```python
from build123d import *

# Parameters (mm, degrees)
F0_R     = 34.5
F1_DEPTH = 1
F2_R     = 34.5
F2_R_2   = 33.5
F3_DEPTH = 18
F4_R     = 40.5
F4_R_2   = 34.5
F4_R_3   = 33.5
F5_DEPTH = 1
F6_SIZE  = 0.99999
F7_R     = 2.5
F8_DEPTH = 25


# Not quite as in the source:
# - a fillet or chamfer is up to 0.001 mm smaller than in the source, because OpenCascade refuses the exact size


with BuildPart() as f1:
    # F0 (on Top) → F1 (new body)
    with BuildSketch(Plane.XY):
        Circle(F0_R)
    extrude(amount=F1_DEPTH)

    # F2 (on face) → F3 (join)
    with BuildSketch(Plane.XY.offset(1)):
        Circle(F2_R)
        Circle(F2_R_2, mode=Mode.SUBTRACT)
    extrude(amount=F3_DEPTH)

    # F4 (on face) → F5 (join)
    with BuildSketch(Plane.XY.offset(19)):
        Circle(F4_R)
        Circle(F4_R_2, mode=Mode.SUBTRACT)
        Circle(F4_R_2)
        Circle(F4_R_3, mode=Mode.SUBTRACT)
    extrude(amount=F5_DEPTH)

    # F6 (size 1 in the source; OpenCascade refuses exactly that, so slightly less here)
    f6_edges = [f1.edges().sort_by_distance(p)[0] for p in [
        (-33.5, 0, 1),
        (-34.5, 0, 0),
        (-33.5, 0, 20),
        (-40.5, 0, 20),
    ]]
    chamfer(f6_edges, length=F6_SIZE)


with BuildPart() as f8:
    # F7 (on Top) → F8 (new body)
    with BuildSketch(Plane.XY):
        with Locations((0, -33.4984026849)):
            Circle(F7_R)
    extrude(amount=F8_DEPTH)


with BuildPart() as f1_1:
    add(f1.part)

    # F9: cut F8
    add(f8.part, mode=Mode.SUBTRACT)


solid = f1_1.part
```
Work out the finished part from the listing and answer in its coordinate system (mm). Round coordinates to 2 decimals unless told otherwise and drop trailing zeros. Loops run counter-clockwise (first coordinate to the right, second up) from the corner with the lowest first, then second, coordinate; pieces in that order, holes last.
(1) The part is cut by section B-B, the plane z = 16.5. Give the vertices of the cut face in (x, y), and give its area (3 significant figures).
Computed values:
outline: (-2.5, -33.41) arc R33.5 cw (long way) to (2.5, -33.41) arc R2.5 cw to (2.32, -34.42) arc R34.5 ccw (long way) to (-2.32, -34.42) arc R2.5 cw to start
area: 209 mm2
(2) Find the intervals of material crossed by L1, parallel to X at y = 0, z = 13.5; L2, parallel to Y at x = 0, z = 11; L3, parallel to X at y = -27.5, z = 8.5, in increasing order.
Computed values:
L1: x = -34.5 to -33.5, 33.5 to 34.5
L2: y = 33.5 to 34.5
L3: x = -20.83 to -19.13, 19.13 to 20.83
(3) Each of these flat-tipped pins is pushed along its axis until it touches: P1, Ø1, axis at x = -0.5, z = 8.5, coming from the +Y side; P2, Ø8, axis at x = 13, z = 14.5, coming from the -Y side; P3, Ø1.5, axis at y = -16, z = 5.5, coming from the +X side. Where does it stop, or does it pass through?
Computed values:
P1: stops at y = 34.5
P2: stops at y = -33.31
P3: stops at x = 30.95
(4) The mould has two halves that part along Y. Classify faces 1 (the conical face through (1.45, 33.63, 0.16)), 2 (the flat face through (0, 0, 1)), 3 (the flat face through (18, -30, 19)): pulls with the +Y half, pulls with the -Y half, needs draft (parallel to the pull), parting line crosses it, or undercut.
Computed values:
face 1: parting line crosses it
face 2: undercut
face 3: needs draft
